Design review of the part shown in the three views and the two pictorial views. Dimensions are in mm from the part's minimum x, y and z. A direction names the side the tool comes from. Give positions to 0.01 mm unless a question says otherwise; leave off trailing zeros. Loops run counter-clockwise (first coordinate to the right, second up) from the corner with the lowest first, then second, coordinate; pieces in that order, holes last. Notation, with made-up numbers: (35, -5) - (68, -5) arc R10 cw to (68, 8) - close; hole circle Ø4 at (8, -12). An arc over 180 degrees is marked (long way). Answer as a JSON object with one key per item and string values.
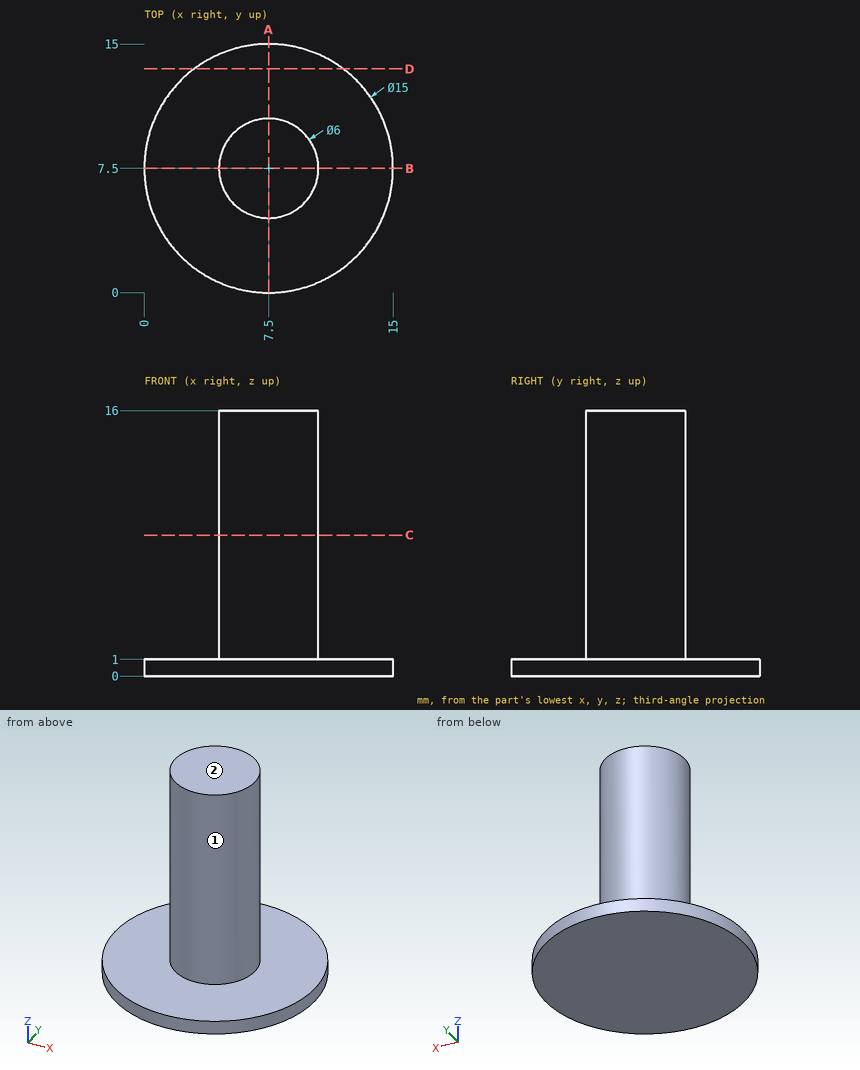
Q1. Consider section A-A, the plane x = 7.5. State the section outline as (y, z) points.
Results:
{"outline": "(0, 0) - (15, 0) - (15, 1) - (10.5, 1) - (10.5, 16) - (4.5, 16) - (4.5, 1) - (0, 1) - close"}
Q2. Consider section D-D, the plane y = 13.5. State the section outline as (x, z) points.
Results:
{"outline": "(3, 0) - (12, 0) - (12, 1) - (3, 1) - close"}
Q3. Clearance check with flat-ended pins moving along their axes: pin 1 Ø1 at (y, z) = (2.5, 9.5) entering from +X; pin 2 Ø1 at (x, y) = (3, 2) entering from +Z. State where each tip first meets the part, or that it passes through.
Results:
{"pin 1": "passes through", "pin 2": "stops at z = 1"}
Q4. Consider section C-C, the plane z = 8.5. State the section outline as (x, y) points, plus the area to 3 significant figures.
Results:
{"outline": "circle Ø6 at (7.5, 7.5)", "area": "28.3 mm^2"}
Q5. To check wall thickness, follow probe 1 along Z at (x, y) = (7.25, 3.25); probe 2 along X at (y, z) = (9.25, 10.5); probe 3 along Y at (x, z) = (7, 9.25). State the ranges of each line that lie inside material, in increasing order. Write a range as [from, to].
Results:
{"probe 1": "z = [0, 1]", "probe 2": "x = [5.06, 9.94]", "probe 3": "y = [4.54, 10.46]"}
Q6. For the marked faces 1 and 2, list the 3-axis set-ups (+Z, -Z, +X, -X, +Y, -Y) from which the entire face can be reached by the end or side of a thin tool; tool diameter is ignored.
Results:
{"face 1": "+Z", "face 2": "+Z, +X, -X, +Y, -Y"}
